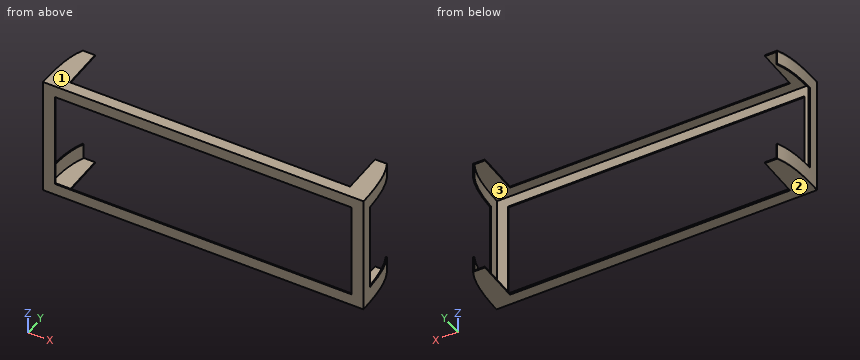
```python
from build123d import *

# Parameters (mm, degrees)
EXTRUDE_THIN2_START    = -127
EXTRUDE_THIN2_DEPTH    = 254
SPLIT1_SURFACE_1_BACK  = 741.713
SPLIT1_SURFACE_1_DEPTH = 1483.426
BOSS_EXTRUDE2_DEPTH    = 2.54
BOSS_EXTRUDE3_DEPTH    = 2.54
SPLIT2_SURFACE_2_BACK  = 743.47
SPLIT2_SURFACE_2_DEPTH = 1486.94


# Read off the part's stored shape, not the designer's step: Extrude-Thin2
with BuildPart() as part:
    # Extrude-Thin2 outline → Extrude-Thin2 (new body)
    with BuildSketch(Plane.XY.offset(EXTRUDE_THIN2_START)):
        with BuildLine():
            Line((-325.542449195, 166.687822519), (-325.542449195, 166.669160537))
            Line((-325.542449195, 166.669160537), (-325.579794085, 166.687822519))
            add(Edge.make_bspline(
                [(-343.046678298, 50.863822519), (-342.854742326, 95.850869045), (-340.503085509, 136.824505781), (-325.579794085, 166.687822519)],
                knots=[0.396009693, 0.396009693, 0.396009693, 0.396009693, 0.524743478, 0.524743478, 0.524743478, 0.524743478], degree=3))
            Line((-343.046678298, 50.863822519), (343.046678298, 50.863822519))
            add(Edge.make_bspline(
                [(325.579794084, 166.687822519), (340.503085509, 136.824505781), (342.854742326, 95.850869045), (343.046678298, 50.863822519)],
                knots=[0.396009693, 0.396009693, 0.396009693, 0.396009693, 0.524743478, 0.524743478, 0.524743478, 0.524743478], degree=3))
            Line((325.579794084, 166.687822519), (323.307694442, 165.552409283))
            add(Edge.make_bspline(
                [(323.307694442, 165.552409283), (326.877593275, 158.408608594), (329.727019011, 150.576977672), (334.257221566, 133.733582984), (335.93764666, 124.722865717), (339.652297398, 96.250136339), (340.357498858, 75.350575466), (340.493401884, 53.403822519)],
                knots=[0, 0, 0, 0, 0.25, 0.25, 0.5, 0.5, 1, 1, 1, 1], degree=3))
            Line((340.493401884, 53.403822519), (-340.493401884, 53.403822519))
            add(Edge.make_bspline(
                [(-340.493401884, 53.403822519), (-340.357498858, 75.350575466), (-339.652297398, 96.250136339), (-335.937646661, 124.722865717), (-334.257221567, 133.733582984), (-329.727019012, 150.576977672), (-326.877593276, 158.408608594), (-323.307694443, 165.552409283)],
                knots=[0, 0, 0, 0, 0.5, 0.5, 0.75, 0.75, 1, 1, 1, 1], degree=3))
            Line((-323.307694443, 165.552409283), (-325.502746425, 166.649320276))
            Line((-325.502746425, 166.649320276), (-325.502746425, 166.687822519))
            Line((-325.502746425, 166.687822519), (-325.542449195, 166.687822519))
        make_face()
    extrude(amount=EXTRUDE_THIN2_DEPTH)

    # Split1: cut with a surface, the side behind it stays
    # Split1 surface: a surface, the sketch's curves swept straight by 1483.426 mm
    with BuildLine(Plane(origin=(0, 0, 0), x_dir=(0, 0, -1), z_dir=(1, 0, 0)).offset(-SPLIT1_SURFACE_1_BACK), mode=Mode.PRIVATE) as split1_surface_1_path:
        Line((-98.324088945, 166.687822519), (-97.98299712, 76.193733858))
        Line((-97.98299712, 76.193733858), (93.487324748, 76.104761498))
        Line((93.487324748, 76.104761498), (93.541066072, 166.687822519))
        Line((93.541066072, 166.687822519), (-98.324088945, 166.687822519))
    split1_surface_1 = Shell.extrude(split1_surface_1_path.wire(), (1 * SPLIT1_SURFACE_1_DEPTH, 0 * SPLIT1_SURFACE_1_DEPTH, 0 * SPLIT1_SURFACE_1_DEPTH))
    split(bisect_by=split1_surface_1, keep=Keep.BOTTOM)

    # Sketch6 → Boss-Extrude2 (add)
    with BuildSketch(Plane.XY.offset(129.54)):
        with BuildLine():
            Line((343.046678298, 50.863822519), (-343.046678298, 50.863822519))
            add(Edge.make_bspline(
                [(-325.579794085, 166.687822519), (-340.503085509, 136.824505781), (-342.854742326, 95.850869045), (-343.046678298, 50.863822519)],
                knots=[0.396009693, 0.396009693, 0.396009693, 0.396009693, 0.524743478, 0.524743478, 0.524743478, 0.524743478], degree=3))
            Line((-325.579794085, 166.687822519), (-325.542449195, 166.687822519))
            Line((-325.542449195, 166.687822519), (-299.506767133, 166.687822519))
            Line((-299.506767133, 166.687822519), (-299.506767133, 75.23611572))
            Line((-299.506767133, 75.23611572), (300.062358087, 75.23611572))
            Line((300.062358087, 75.23611572), (300.062358087, 166.687822519))
            Line((300.062358087, 166.687822519), (325.579794084, 166.687822519))
            add(Edge.make_bspline(
                [(325.579794084, 166.687822519), (340.503085509, 136.824505781), (342.854742326, 95.850869045), (343.046678298, 50.863822519)],
                knots=[0.396009693, 0.396009693, 0.396009693, 0.396009693, 0.524743478, 0.524743478, 0.524743478, 0.524743478], degree=3))
        make_face()
    extrude(amount=-BOSS_EXTRUDE2_DEPTH)

    # Sketch7 → Boss-Extrude3 (add)
    with BuildSketch(Plane(origin=(0, 0, -129.54), x_dir=(-1, 0, 0), z_dir=(0, 0, -1))):
        with BuildLine():
            Line((0, 50.863822519), (0, 75.23611572))
            Line((0, 75.23611572), (-300.062358087, 75.23611572))
            Line((-300.062358087, 75.23611572), (-300.062358087, 166.687822519))
            Line((-300.062358087, 166.687822519), (-325.502746425, 166.687822519))
            Line((-325.502746425, 166.687822519), (-325.542449195, 166.687822519))
            Line((-325.542449195, 166.687822519), (-325.579794085, 166.687822519))
            add(Edge.make_bspline(
                [(-325.579794085, 166.687822519), (-340.503085509, 136.824505781), (-342.854742326, 95.850869045), (-343.046678298, 50.863822519)],
                knots=[0.396009693, 0.396009693, 0.396009693, 0.396009693, 0.524743478, 0.524743478, 0.524743478, 0.524743478], degree=3))
            Line((-343.046678298, 50.863822519), (0, 50.863822519))
        make_face()
        with BuildLine():
            Line((299.506767133, 75.23611572), (0, 75.23611572))
            Line((0, 75.23611572), (0, 50.863822519))
            Line((0, 50.863822519), (343.046678298, 50.863822519))
            add(Edge.make_bspline(
                [(325.579794084, 166.687822519), (340.503085509, 136.824505781), (342.854742326, 95.850869045), (343.046678298, 50.863822519)],
                knots=[0.396009693, 0.396009693, 0.396009693, 0.396009693, 0.524743478, 0.524743478, 0.524743478, 0.524743478], degree=3))
            Line((325.579794084, 166.687822519), (299.506767133, 166.687822519))
            Line((299.506767133, 166.687822519), (299.506767133, 75.23611572))
        make_face()
    extrude(amount=-BOSS_EXTRUDE3_DEPTH)

    # Split2: cut with a surface, the side it looks to stays
    # Split2 surface: a surface, the sketch's curves swept straight by 1486.94 mm
    with BuildLine(Plane(origin=(0, 0, 0), x_dir=(1, 0, 0), z_dir=(0, 1, 0)).offset(-SPLIT2_SURFACE_2_BACK), mode=Mode.PRIVATE) as split2_surface_2_path:
        Line((-317.646678298, 104.14), (317.080123639, 104.14))
        Line((317.080123639, 104.14), (317.080123639, -104.14))
        Line((317.080123639, -104.14), (-317.646678298, -104.14))
        Line((-317.646678298, -104.14), (-317.646678298, 104.14))
    split2_surface_2 = Shell.extrude(split2_surface_2_path.wire(), (0 * SPLIT2_SURFACE_2_DEPTH, 1 * SPLIT2_SURFACE_2_DEPTH, 0 * SPLIT2_SURFACE_2_DEPTH))
    split(bisect_by=split2_surface_2, keep=Keep.TOP)


solid = part.part
```
CAD build for the part. Positions are in the model's coordinates, mm. Face numbers are marked on the shaded views. Round coordinates to 2 decimals unless told otherwise and drop trailing zeros. Loops run counter-clockwise (first coordinate to the right, second up) from the corner with the lowest first, then second, coordinate; pieces in that order, holes last. Notation, with made-up numbers: (74.5, 7) - (83.5, 7) arc R21 cw to (83.5, 41) - close; hole circle Ø4 at (70.25, -12). An arc over 180 degrees is marked (long way). Return JSON: item names as keys, results as strings. Group by question number.
Q1. Band-saw the part on A-A on x = -185. Give the cut face in (y, z).
Q2. Two-plate mould, pull along Z, no slides. Class the marked faces 1, 2 and 3: +Z half, -Z half, draft (parallel to the pull), parting line (faces both ways), or undercut.
Q3. Band-saw the part on B-B on y = 91. Give the number of separate pieces and of enclosed holes in the cut face, plus the area to 3 significant figures.
Q4. Drill centre lines: line 1 along Z through (x, y) = (29.5, 57.5); line 2 along X through (y, z) = (56, 16); line 3 along X through (y, z) = (61, 80). Where is each one in solid material? Low to high. Write a range as [from, to].
Q5. Flat gauge pins, fed straight in: pin 1 Ø2 at (x, z) = (41, -128.5) entering from +Y; pin 2 Ø3 at (y, z) = (129.5, 128) entering from +X; pin 3 Ø2 at (y, z) = (135.5, -128.5) entering from +X. Where does each tip first touch, or does it go through?
Solutions:
{
 "1": {"outline": "(50.86, -129.54) - (75.24, -129.54) - (75.24, -127) - (53.4, -127) - (53.4, -104.14) - (50.86, -104.14) - close; (50.86, 104.14) - (53.4, 104.14) - (53.4, 127) - (75.24, 127) - (75.24, 129.54) - (50.86, 129.54) - close"},
 "2": {"face 1": "+Z half", "face 2": "-Z half", "face 3": "undercut"},
 "3": {"separate pieces": "4", "enclosed holes": "0", "area": "746 mm^2"},
 "4": {"line 1": "z = [-129.54, -127], [127, 129.54]", "line 2": "x = [-343.01, -340.47], [340.47, 343.01]", "line 3": "x = [-342.96, -340.42], [340.42, 342.96]"},
 "5": {"pin 1": "stops at y = 75.24", "pin 2": "stops at x = 337.76", "pin 3": "stops at x = 336.46"}
}
